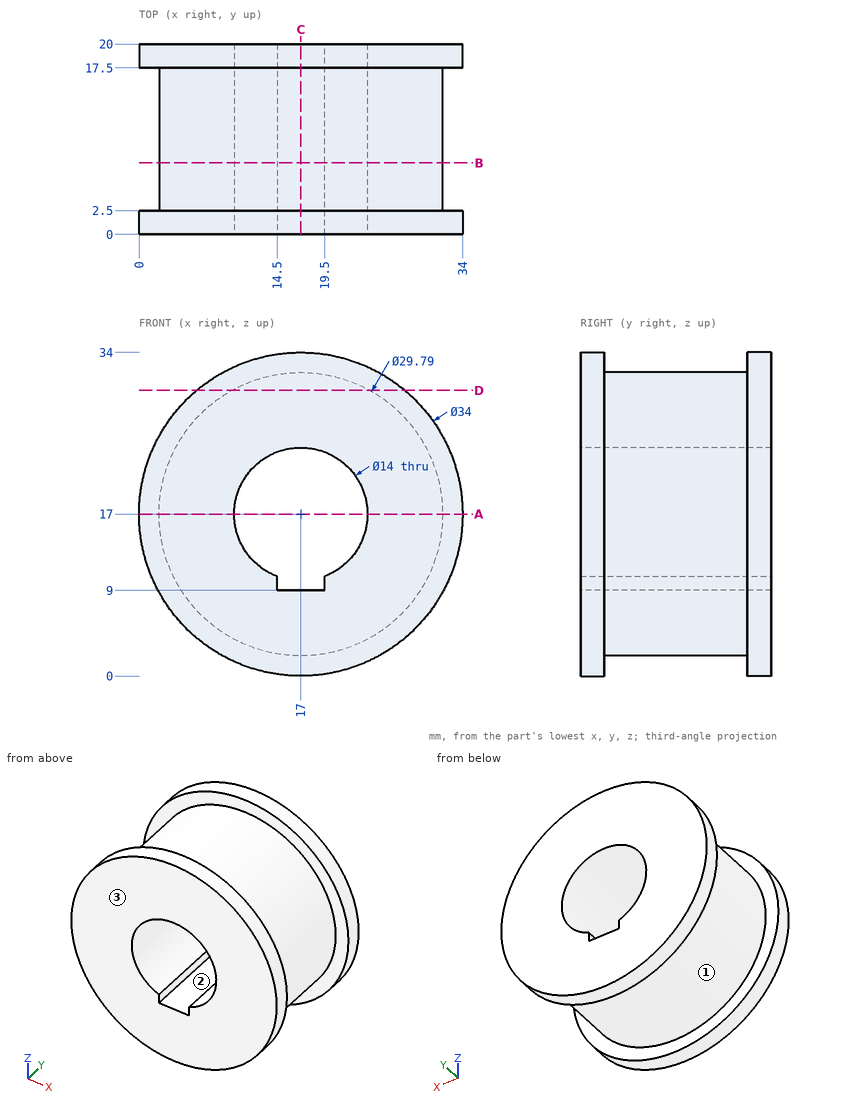
For this review, use the dimensioned drawing (mm, ordinates from the lowest corner) and the shaded views. Give positions to 0.01 mm unless a question says otherwise; leave off trailing zeros. Write each loop counter-clockwise with the first axis right and the second up, starting at its lowest first coordinate (ties: lowest second). Pieces come first, ordered by that corner, then holes. Notation, with made-up numbers: M 9.5,-28.75 L 33.5,-28.75 A4 cw 33.5,-22.75 Z; hole C 48.5,-39.5 d8. An arc over 180 degrees is marked long. Write item = value, one per line. Start each with the question number.
Q1. We need section D-D (z = 30). State the section outline as (x, y) points, plus the area to 3 significant figures.
Q2. For line 1 (Z direction, x = 17, y = 9.5) (3 decimals); line 2 (X direction, y = 4.5, z = 17) (3 decimals); line 3 (Y direction, x = 3.5, z = 27), list the stretches that pass through material, from the lowest coordinate up.
Q3. Mouldability with a two-part tool opening along X and no side actions: class the marked faces 1, 2 and 3 as released by +X, released by -X, zero draft, split by the parting line, or undercut.
Q4. We need section A-A (z = 17). State the section outline as (x, y) points (3 decimals), plus the area to 3 significant figures.
Q5. We need section C-C (x = 17). State the section outline as (y, z) points (3 decimals), plus the area to 3 significant figures.
Q6. We need section B-B (y = 7.5). State the section outline as (x, z) points (3 decimals).
Q7. Clearance check with flat-ended pins moving along their axes: pin 1 (10 mm diameter, centred on x = 13.5, z = 23.5, fed in from -Y); pin 2 (1.2 mm diameter, centred on y = 8.5, z = 9.5, fed in from +X); pin 3 (2 mm diameter, centred on x = 10, y = 2, fed in from +Z); pin 4 (1.5 mm diameter, centred on x = 4, y = 18, fed in from -Z). State where each tip first meets the part, or that it passes through.
Result set:
q1.outline = M 6.05,0 L 27.95,0 L 27.95,2.5 L 24.27,2.5 L 24.27,17.5 L 27.95,17.5 L 27.95,20 L 6.05,20 L 6.05,17.5 L 9.73,17.5 L 9.73,2.5 L 6.05,2.5 Z
q1.area = 328 mm2
q2.line_1 = 2.105 to 9, 24 to 31.895
q2.line_2 = 2.105 to 10, 24 to 31.895
q2.line_3 = 0 to 2.5, 17.5 to 20
q3.face_1 = split by the parting line
q3.face_2 = undercut
q3.face_3 = zero draft
q4.outline = M 0,0 L 10,0 L 10,20 L 0,20 L 0,17.5 L 2.105,17.5 L 2.105,2.5 L 0,2.5 Z; M 24,0 L 34,0 L 34,2.5 L 31.895,2.5 L 31.895,17.5 L 34,17.5 L 34,20 L 24,20 Z
q4.area = 337 mm2
q5.outline = M 0,0 L 2.5,0 L 2.5,2.105 L 17.5,2.105 L 17.5,0 L 20,0 L 20,9 L 0,9 Z; M 0,24 L 20,24 L 20,34 L 17.5,34 L 17.5,31.895 L 2.5,31.895 L 2.5,34 L 0,34 Z
q5.area = 317 mm2
q6.outline = C 17,17 d29.79; hole M 14.5,9 L 19.5,9 L 19.5,10.462 A7 ccw long 14.5,10.462 Z
q7.pin_1 = 0
q7.pin_2 = 30.2
q7.pin_3 = 32.91
q7.pin_4 = 5.21
